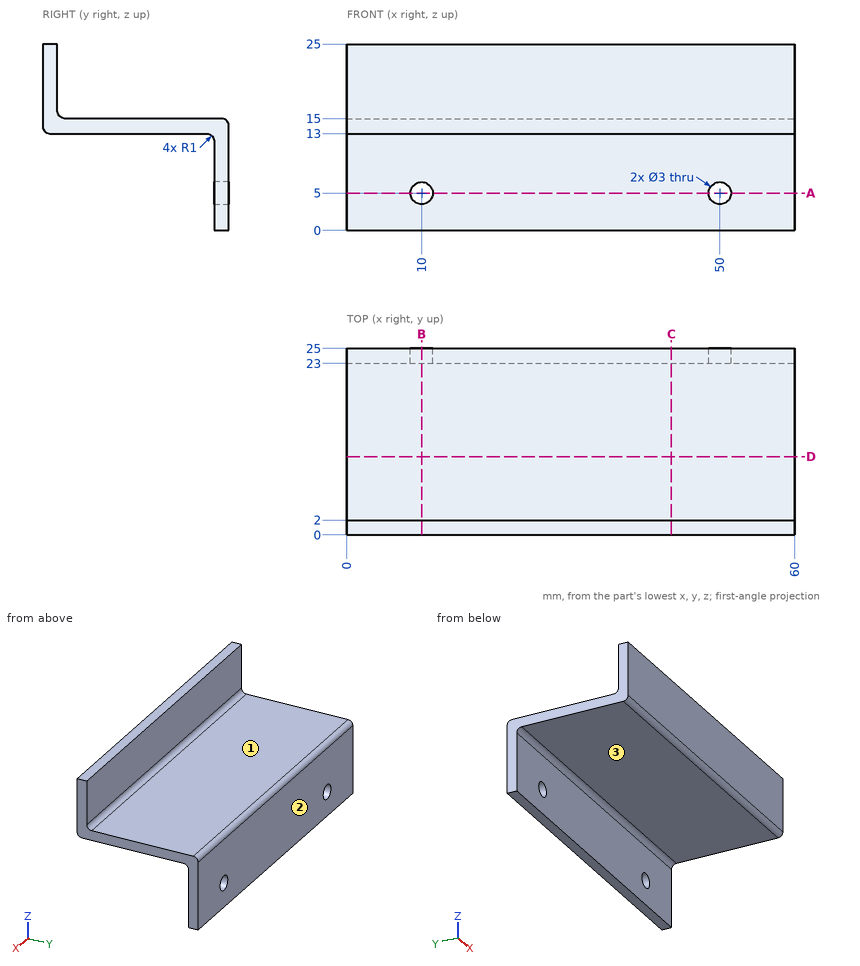
Here's the drawing with two shaded views (mm, measured from the low corner). I have some questions. A direction names the side the tool comes from. Coordinates: 2 decimals unless noted, no trailing zeros. Order: outer loops, then holes, each group sorted by start corner. A loop starts at its lowest first (then second) coordinate and runs counter-clockwise, first axis right, second up.
Q1. Will these pins go through, and if not, where does the flat tip stop? pin 1 (5 mm diameter, centred on y = 22, z = 3.5, fed in from -X); pin 2 (13 mm diameter, centred on x = 29.5, z = 3, fed in from -Y); pin 3 (10.5 mm diameter, centred on x = 17, y = 14, fed in from +Z); pin 4 (1.5 mm diameter, centred on x = 37, y = 4, fed in from -Z).
Q2. Please list where these lines run through material, in increasing order: L1, parallel to X at y = 24.45, z = 5; L2, parallel to Z at x = 46.5, y = 7.25; L3, parallel to Y at x = 10.5, z = 9.5.
Q3. Suppose I cut it at B-B on x = 10. Please give me the cut outline in (y, z).
Q4. Suppose I cut it at C-C on x = 43.5. Please give me the cut outline in (y, z).
Q5. Suppose I cut it at D-D on y = 10.5. Please give me the cut outline in (x, z).
Q6. Suppose I cut it at A-A on z = 5. Please give me the cut outline in (x, y), and give its area (3 significant figures).
Q7. Which directions (+Z, -Z, +X, -X, +Y, -Y) give clear straight access to the entire face, cutting with the end or side of a thin tool? Please do the marked faces 1, 2 and 3.
Answer:
1. pin 1: stops at x = 0
1. pin 2: stops at y = 23
1. pin 3: stops at z = 15
1. pin 4: stops at z = 13
2. L1: x = 0 to 8.5, 11.5 to 48.5, 51.5 to 60
2. L2: z = 13 to 15
2. L3: y = 23 to 25
3. outline: (0, 14) arc R1 ccw to (1, 13) - (22, 13) arc R1 cw to (23, 12) - (23, 6.5) - (25, 6.5) - (25, 14) arc R1 ccw to (24, 15) - (3, 15) arc R1 cw to (2, 16) - (2, 25) - (0, 25) - close; (23, 0) - (25, 0) - (25, 3.5) - (23, 3.5) - close
4. outline: (0, 14) arc R1 ccw to (1, 13) - (22, 13) arc R1 cw to (23, 12) - (23, 0) - (25, 0) - (25, 14) arc R1 ccw to (24, 15) - (3, 15) arc R1 cw to (2, 16) - (2, 25) - (0, 25) - close
5. outline: (0, 13) - (60, 13) - (60, 15) - (0, 15) - close
6. outline: (0, 23) - (8.5, 23) - (8.5, 25) - (0, 25) - close; (11.5, 23) - (48.5, 23) - (48.5, 25) - (11.5, 25) - close; (51.5, 23) - (60, 23) - (60, 25) - (51.5, 25) - close
6. area: 108 mm2
7. face 1: +Z, +X, -X, +Y
7. face 2: +Z, -Z, +X, -X, +Y
7. face 3: -Z, +X, -X, -Y
